Could you check a few things on this model? Use its own coordinates, in mm. Coordinates: 2 decimals unless noted, no trailing zeros. Write each loop counter-clockwise with the first axis right and the second up, starting at its lowest first coordinate (ties: lowest second). Pieces come first, ordered by that corner, then holes. Notation, with made-up numbers: M 71,48.25 L 96,48.25 A31 cw 96,84.25 Z; hole C 58.25,9.5 d9. An arc over 180 degrees is marked long. Write item = value, one per line.
```python
from build123d import *

# Parameters (mm, degrees)
BOSS_EXTRUDE1_DEPTH = 15
BOSS_EXTRUDE2_DEPTH = 2.5
SKETCH3_R           = 2
BOSS_EXTRUDE3_DEPTH = 15


with BuildPart() as part:
    # Sketch1 → Boss-Extrude1 (new, symmetric)
    with BuildSketch(Plane.XY):
        Polygon((-66, 10.962277833), (-1, 13.462277833), (-1, 18.465974691), (-71, 15.773666999), (-71, -1), (-66, -1), align=None)
    extrude(amount=BOSS_EXTRUDE1_DEPTH, both=True)

    # Sketch2 → Boss-Extrude2 (add, symmetric)
    with BuildSketch(Plane.XY):
        with BuildLine():
            Line((-68.329320747, 15.876385432), (-68.49608066, 20.212143147))
            add(Edge.make_bspline(
                [(-68.49608066, 20.212143147), (-58.446239367, 154.187541724), (-107.856515034, 229.820456607), (2.961147934, 154.665009331)],
                knots=[0, 0, 0, 0, 1, 1, 1, 1], degree=3))
            Line((2.961147934, 154.665009331), (-55.159919487, 16.382900865))
            Line((-55.159919487, 16.382900865), (-68.329320747, 15.876385432))
        make_face()
    extrude(amount=BOSS_EXTRUDE2_DEPTH, both=True)

    # Sketch3 → Boss-Extrude3 (add)
    with BuildSketch(Plane(origin=(0, 0, -2.5), x_dir=(-1, 0, 0), z_dir=(0, 0, -1))):
        with Locations((49.038852066, 172.382900865)):
            Circle(SKETCH3_R)
    extrude(amount=BOSS_EXTRUDE3_DEPTH)


solid = part.part
```
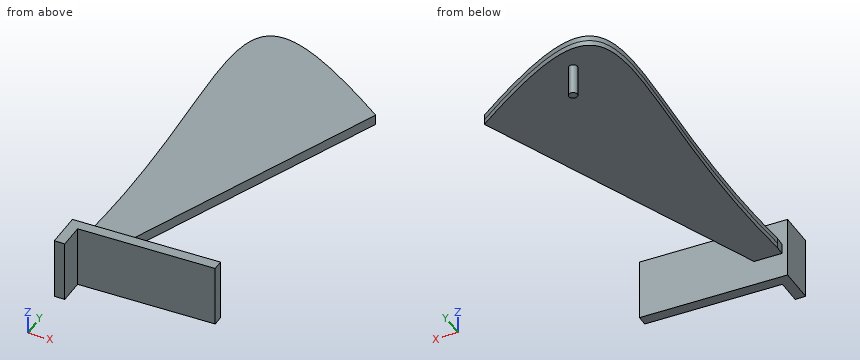
Item 1: Imagine slicing it at A-A (z = 8.5). Write out the boundary of the cut face in (x, y).
Numbers:
outline = M -71,-1 L -66,-1 L -66,10.96 L -1,13.46 L -1,18.47 L -71,15.77 Z
Item 2: If I drill on line 1 along Z through (x, y) = (-26, 124); line 2 along X through (y, z) = (14.5, 10.5); line 3 along Y through (x, z) = (-52.5, -2), over which ranges is the centre line in solid material (lowest first)?
Numbers:
line_1 = -2.5 to 2.5
line_2 = -71 to -1
line_3 = 11.48 to 16.49, 22.71 to 184.05
Item 3: Imagine slicing it at B-B (z = -9). Write out the boundary of the cut face in (x, y).
Numbers:
outline = M -71,-1 L -66,-1 L -66,10.96 L -1,13.46 L -1,18.47 L -71,15.77 Z; C -49.04,172.38 d4
Item 4: I'm going to push flat-ended pins straight in: P1, Ø22, axis at x = -51, y = 103, coming from the +Z side; P2, Ø12, axis at x = -8, z = -8, coming from the +Y side; P3, Ø1.5, axis at y = 15.5, z = 4, coming from the +X side. Where does each tip first touch, or does it pass through?
Numbers:
P1 = 2.5
P2 = 163.49
P3 = -1
